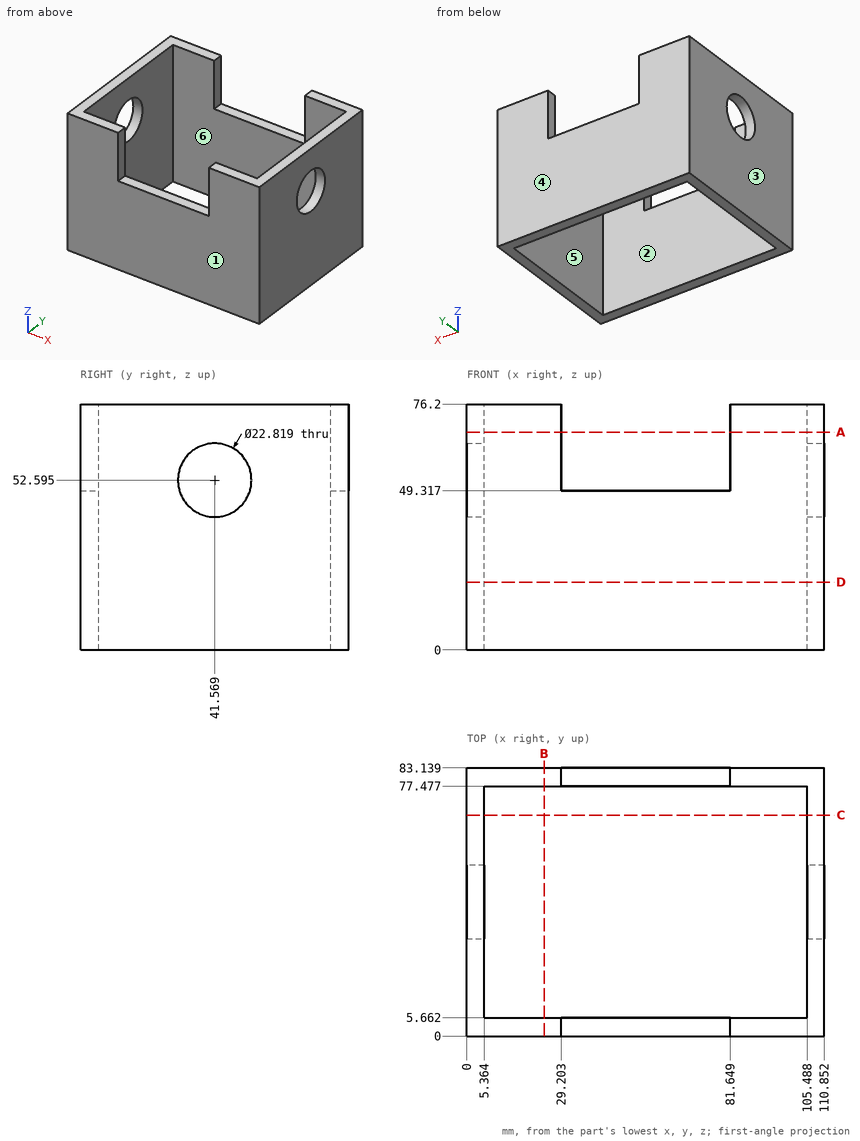
Can you work these out from the drawing? Everything is in mm from the part's minimum corner. A direction names the side the tool comes from. Coordinates: 2 decimals unless noted, no trailing zeros. Loops run counter-clockwise (first coordinate to the right, second up) from the corner with the lowest first, then second, coordinate; pieces in that order, holes last.
1) Imagine slicing it at B-B on x = 24. List the corners of the cut face in (y, z) for me.
2) Imagine slicing it at C-C on y = 68.5. List the corners of the cut face in (x, z) for me.
3) For pin 1 (3 mm diameter, centred on y = 25, z = 25.5, fed in from -X); pin 2 (6 mm diameter, centred on x = 69.5, z = 53.5, fed in from -Y); pin 3 (3 mm diameter, centred on x = 45.5, y = 80.5, fed in from +Z), each with a flat end and sliding along its axis, tell me the tip position at first contact or that it passes through.
4) Which directions (+Z, -Z, +X, -X, +Y, -Y) give clear straight access to the entire face, cutting with the end or side of a thin tool? Please do the marked faces 1 and 2.
5) Imagine slicing it at A-A on z = 67.5. List the corners of the cut face in (x, y) for me.
6) I need wall thicknesses on probe 1 along X at (y, z) = (17, 55.5); probe 2 along Y at (x, z) = (48, 28); probe 3 along X at (y, z) = (78, 67.5). Which ranges of each line are inside material? Lowest first, please.
7) Imagine slicing it at D-D on z = 21. List the corners of the cut face in (x, y) for me.
8) Thinking about a two-plate mould opening in X: for the marked faces 3, 4, 5 and 6, which applies, pulls with the +X half, pulls with the -X half, needs draft (parallel to the pull), parting line crosses it, or undercut?
Completed:
1. outline: (0, 0) - (5.66, 0) - (5.66, 76.2) - (0, 76.2) - close; (77.48, 0) - (83.14, 0) - (83.14, 76.2) - (77.48, 76.2) - close
2. outline: (0, 0) - (5.36, 0) - (5.36, 76.2) - (0, 76.2) - close; (105.49, 0) - (110.85, 0) - (110.85, 76.2) - (105.49, 76.2) - close
3. pin 1: stops at x = 0
3. pin 2: passes through
3. pin 3: stops at z = 49.32
4. face 1: +Z, -Z, +X, -X, -Y
4. face 2: +Z, -Z
5. outline: (0, 0) - (29.2, 0) - (29.2, 5.66) - (5.36, 5.66) - (5.36, 77.48) - (29.2, 77.48) - (29.2, 83.14) - (0, 83.14) - close; (81.65, 0) - (110.85, 0) - (110.85, 83.14) - (81.65, 83.14) - (81.65, 77.48) - (105.49, 77.48) - (105.49, 5.66) - (81.65, 5.66) - close
6. probe 1: x = 0 to 5.36, 105.49 to 110.85
6. probe 2: y = 0 to 5.66, 77.48 to 83.14
6. probe 3: x = 0 to 29.2, 81.65 to 110.85
7. outline: (0, 0) - (110.85, 0) - (110.85, 83.14) - (0, 83.14) - close; hole (5.36, 5.66) - (105.49, 5.66) - (105.49, 77.48) - (5.36, 77.48) - close
8. face 3: pulls with the -X half
8. face 4: needs draft
8. face 5: undercut
8. face 6: undercut
